```python
from build123d import *

# Parameters (mm, degrees)
EXTRUDE_1_DEPTH = 10
FILLET_1_R      = 2


with BuildPart() as part:
    # 草图1 → 凸台-拉伸1 (new body)
    with BuildSketch(Plane(origin=(0, 0, 0), x_dir=(1, 0, 0), z_dir=(0, 1, 0))):
        Polygon((-15, -175), (-15, -155), (5, -155), (5, -157), (15, -155), (15, -152), (-15, -152), (-15, 152), (15, 152), (15, 155), (5, 157), (5, 155), (-15, 155), (-15, 175), (5, 175), (5, 173), (15, 175), (15, 178), (-24.323280296, 178), (-85, -138), (-20, -138), (-20, -178), (15, -178), (15, -175), (5, -173), (5, -175), align=None)
        Polygon((-20, 174), (-20, -133), (-78.948585282, -133), align=None, mode=Mode.SUBTRACT)
    extrude(amount=EXTRUDE_1_DEPTH)

    # 圆角1
    fillet_1_edges = [part.edges().sort_by_distance(p)[0] for p in [
        (-24.323280296, 5, -178),
        (-85, 5, 138),
        (-20, 5, 178),
        (15, 5, 175),
        (15, 5, -155),
        (15, 5, -175),
        (-20, 5, -174),
        (-20, 5, 133),
        (-78.948585282, 5, 133),
        (15, 5, 155),
    ]]
    fillet(fillet_1_edges, radius=FILLET_1_R)


solid = part.part
```
Design review of the part built by this model. Coordinates are the model's own, in mm. A direction names the side the tool comes from. Give positions to 0.01 mm unless a question says otherwise; leave off trailing zeros. Order: outer loops, then holes, each group sorted by start corner. A loop starts at its lowest first (then second) coordinate and runs counter-clockwise, first axis right, second up. Notation, with made-up numbers: (64, 55) - (116, 55) arc R19 cw to (116, 67) - close; hole circle Ø11 at (81.5, 88). An arc over 180 degrees is marked (long way). Use a Markdown table: item, result. Add a question column.
(1) Add section C-C on z = 141. Give the boundary of the cut face in (x, y).
(2) Clearance check with flat-ended pins moving along their axes: P1, Ø1.6, axis at y = 6, z = -156.5, coming from the -X side; P2, Ø0.6, axis at y = 5, z = 174, coming from the -X side; P3, Ø5, axis at y = 4.5, z = -28, coming from the -X side. State where each tip first meets the part, or that it passes through.
(3) Add section B-B on x = -40.5. Give the boundary of the cut face in (y, z), then the cut area to 3 significant figures.
(4) Wall thickness on probe 1 along Z at (x, y) = (-4.5, 5.25); probe 2 along Z at (x, y) = (-21.5, 8.5); probe 3 along Z at (x, y) = (5.5, 2.75): over which ranges is each line inside the solid? List them lowest first. Write a range as [from, to].
(5) Add section A-A on z = 81. Give the boundary of the cut face in (x, y), then the cut area to 3 significant figures.
(6) Machinability: for faces 1 (the face through (-52, 5, 138)), 2 (the face through (9.14, 4.93, -173.83)), 3 (the face through (-49, 5, 133)), which of the approach directions +Z, -Z, +X, -X, +Y, -Y give a long, thin tool a straight path to every point of the face, cutting with its end or side? Answer none if there is none.
(7) Mouldability with a two-part tool opening along X and no side actions: class faces 4 (the face through (0, 5, 152)), 5 (the face through (-5, 5, 175)), 6 (the face through (-15, 5, 2)) as +X half, -X half, draft (parallel to the pull), parting line (faces both ways), or undercut.
Report:
| question | item | result |
|---|---|---|
| 1 | outline | (-20, 0) - (-15, 0) - (-15, 10) - (-20, 10) - close |
| 2 | P1 | stops at x = -28.61 |
| 2 | P2 | stops at x = -20 |
| 2 | P3 | stops at x = -53.61 |
| 3 | outline | (0, -93.75) - (10, -93.75) - (10, -67.24) - (0, -67.24) - close; (0, 133) - (10, 133) - (10, 138) - (0, 138) - close |
| 3 | area | 315 mm² |
| 4 | probe 1 | z = [-178, -175], [-155, -152], [152, 155], [175, 178] |
| 4 | probe 2 | z = [-178, -154.91], [132.94, 138] |
| 4 | probe 3 | z = [-178, -173.1], [-156.9, -152], [152, 156.9], [173.1, 178] |
| 5 | outline | (-74.06, 0) - (-68.96, 0) - (-68.96, 10) - (-74.06, 10) - close; (-20, 0) - (-15, 0) - (-15, 10) - (-20, 10) - close |
| 5 | area | 101 mm² |
| 6 | face 1 | +Z, -X, +Y, -Y |
| 6 | face 2 | +X, +Y, -Y |
| 6 | face 3 | +Y, -Y |
| 7 | face 4 | draft |
| 7 | face 5 | undercut |
| 7 | face 6 | +X half |
